Verification items for this drawing (mm, ordinates from the low corner). A direction names the side the tool comes from. Round coordinates to 2 decimals unless told otherwise and drop trailing zeros. Loops run counter-clockwise (first coordinate to the right, second up) from the corner with the lowest first, then second, coordinate; pieces in that order, holes last. Notation, with made-up numbers: M -26.5,-12 L 30.5,-12 A24 cw 30.5,12 Z; hole C -18.75,67.5 d5. An arc over 180 degrees is marked long. One line per item, written item: value.
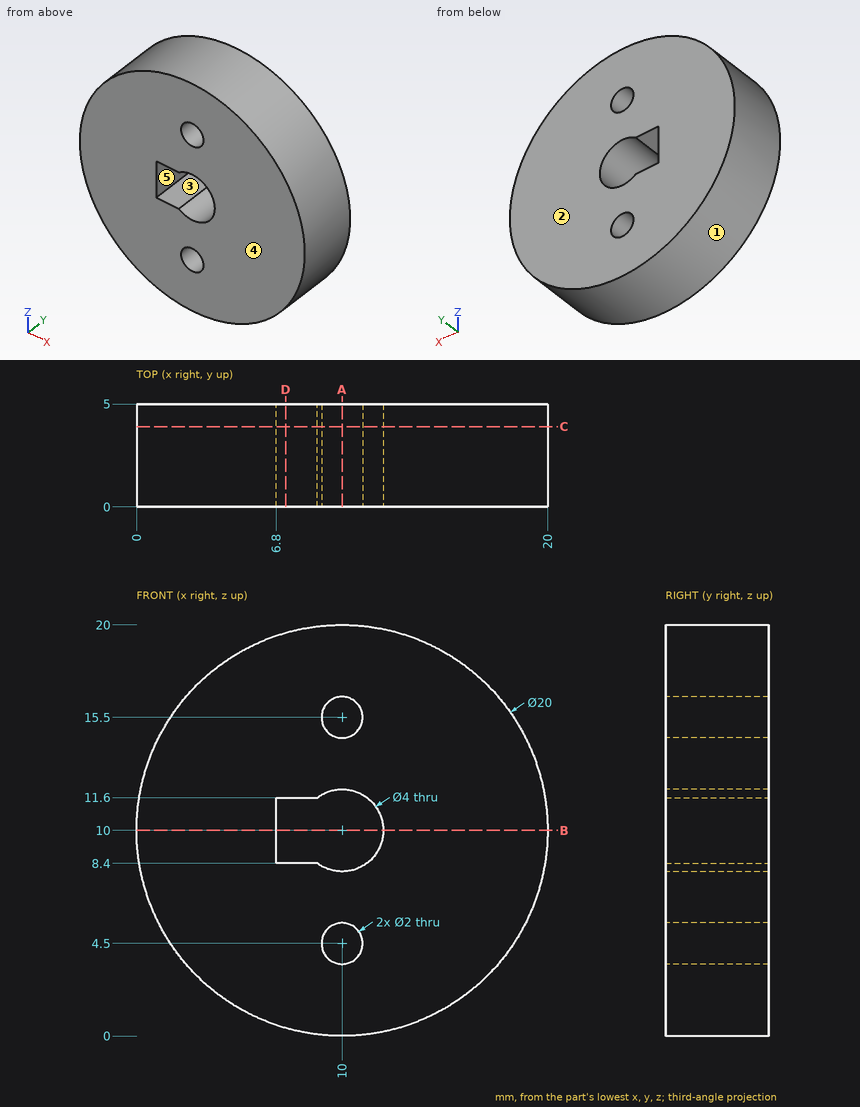
(1) Depth check by flat-ended pin: pin 1 Ø1.6 at (x, y) = (7.5, 3) entering from +Z; pin 2 Ø1.5 at (x, z) = (16, 10) entering from -Y; pin 3 Ø2 at (x, y) = (7.5, 2) entering from -Z; pin 4 Ø1.5 at (y, z) = (4, 11.5) entering from +X. Enter the tip coordinate at first touch or a pass-through.
Completed:
pin 1: stops at z = 19.85
pin 2: stops at y = 0
pin 3: stops at z = 0.11
pin 4: stops at x = 19.97
(2) Tool access check on the marked faces 4 and 5. Record the directions out of +Z, -Z, +X, -X, +Y, -Y that give a thin tool (end or side, any length) a straight path to the whole face; none if there is none.
Completed:
face 4: +Z, -Z, +X, -X, -Y
face 5: +Y, -Y
(3) Sectioned sample at A-A on x = 10. Enter the section's corners in (y, z).
Completed:
outline: M 0,0 L 5,0 L 5,3.5 L 0,3.5 Z; M 0,5.5 L 5,5.5 L 5,8 L 0,8 Z; M 0,12 L 5,12 L 5,14.5 L 0,14.5 Z; M 0,16.5 L 5,16.5 L 5,20 L 0,20 Z
(4) Sectioned sample at B-B on z = 10. Enter the section's corners in (x, y), and give its area (3 significant figures).
Completed:
outline: M 0,0 L 6.8,0 L 6.8,5 L 0,5 Z; M 12,0 L 20,0 L 20,5 L 12,5 Z
area: 74.0 mm^2
(5) Thickness scan on L1, parallel to X at y = 3.75, z = 3.75; L2, parallel to X at y = 2.55, z = 11; L3, parallel to Z at x = 7.25, y = 4.5. Record the ranges inside material, lowest first. Write a range as from..to.
Completed:
L1: x = 2.19..9.34, 10.66..17.81
L2: x = 0.05..6.8, 11.73..19.95
L3: z = 0.39..8.4, 11.6..19.61
(6) Sectioned sample at C-C on y = 3.9. Enter the section's corners in (x, z).
Completed:
outline: C 10,10 d20; hole M 6.8,8.4 L 8.8,8.4 A2 ccw long 8.8,11.6 L 6.8,11.6 Z; hole C 10,4.5 d2; hole C 10,15.5 d2
(7) Sectioned sample at D-D on x = 7.25. Enter the section's corners in (y, z), and give its area (3 significant figures).
Completed:
outline: M 0,0.39 L 5,0.39 L 5,8.4 L 0,8.4 Z; M 0,11.6 L 5,11.6 L 5,19.61 L 0,19.61 Z
area: 80.1 mm^2
(8) Mould release check, pull along X, two halves, no side actions. Record for the marked faces 1, 2 and 3: +X half, -X half, draft (parallel to the pull), parting line (faces both ways), or undercut.
Completed:
face 1: parting line
face 2: draft
face 3: undercut
